Input: dimensioned drawing with shaded views. Units: mm. Origin: part minimum x, y, z. Coordinates: 2 decimals unless noted, no trailing zeros. Order: outer loops, then holes, each group sorted by start corner. A loop starts at its lowest first (then second) coordinate and runs counter-clockwise, first axis right, second up. Notation, with made-up numbers: (87, 61) -> (103, 61) arc R22 cw to (103, 84) -> close; hole circle Ø9 at (41.25, 58). An arc over 180 degrees is marked (long way). Answer as CSV lines item,"result".
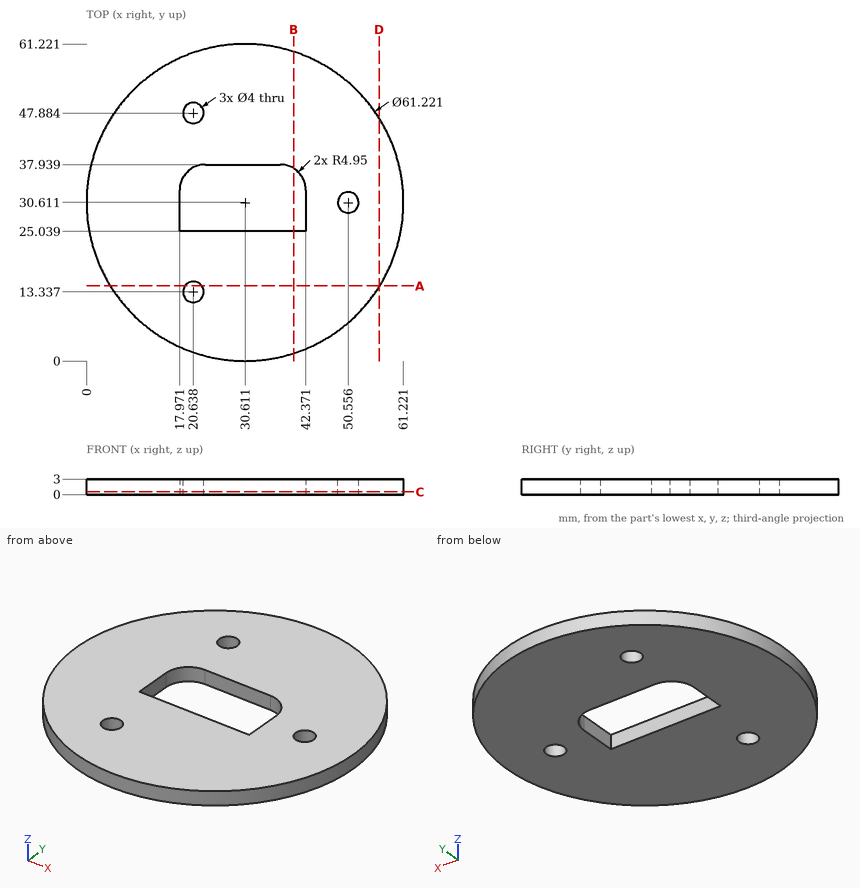
1. Ray query, line 1 along X through (y, z) = (32, 2.55) (1 decimal); line 2 along Y through (x, z) = (30.5, 1.25); line 3 along X through (y, z) = (47, 0.45) (1 decimal). Return the intervals inside material, ascending.
Findings:
line 1,"x = 0 to 18, 42.4 to 49.1, 52 to 61.2"
line 2,"y = 0 to 25.04, 37.94 to 61.22"
line 3,"x = 4.8 to 18.8, 22.4 to 56.5"
2. Cut plane D-D (x = 56.5). Return the cut outline in (y, z).
Findings:
outline,"(14.28, 0) -> (46.94, 0) -> (46.94, 3) -> (14.28, 3) -> close"
3. Cut plane C-C (z = 0.5). Return the cut outline in (x, y).
Findings:
outline,"circle Ø61.22 at (30.61, 30.61); hole (17.97, 25.04) -> (42.37, 25.04) -> (42.37, 32.99) arc R4.95 ccw to (37.42, 37.94) -> (22.92, 37.94) arc R4.95 ccw to (17.97, 32.99) -> close; hole circle Ø4 at (20.64, 13.34); hole circle Ø4 at (20.64, 47.88); hole circle Ø4 at (50.56, 30.61)"
4. Cut plane B-B (x = 40). Return the cut outline in (y, z) (1 decimal), plus the area to 3 significant figures.
Findings:
outline,"(1.5, 0) -> (25, 0) -> (25, 3) -> (1.5, 3) -> close; (37.2, 0) -> (59.7, 0) -> (59.7, 3) -> (37.2, 3) -> close"
area,"138 mm2"
5. Contact query for flat-ended pins moving along their axis: pin 1 (1.5 mm diameter, centred on y = 31, z = 1.5, fed in from -X); pin 2 (1 mm diameter, centred on x = 47, z = 2, fed in from -Y); pin 3 (0.9 mm diameter, centred on x = 26.5, z = 1, fed in from +Y). Output: stop coordinate, or through.
Findings:
pin 1,"stops at x = 0"
pin 2,"stops at y = 4.45"
pin 3,"stops at y = 61"
6. Cut plane A-A (y = 14.5). Return the cut outline in (x, z) (1 decimal).
Findings:
outline,"(4.6, 0) -> (19, 0) -> (19, 3) -> (4.6, 3) -> close; (22.3, 0) -> (56.6, 0) -> (56.6, 3) -> (22.3, 3) -> close"
